Could you check a few things on this model? Use its own coordinates, in mm. A direction names the side the tool comes from. Coordinates: 2 decimals unless noted, no trailing zeros. Loops run counter-clockwise (first coordinate to the right, second up) from the corner with the lowest first, then second, coordinate; pieces in that order, holes last. Notation, with made-up numbers: (-3, 10) - (12, 10) arc R20 cw to (12, 18) - close; hole circle Ø4 at (4.25, 4). An arc over 180 degrees is marked (long way). One line per item, written item: value. Start each with the question number.
(1) If we section it at C-C on y = -6.75: Write out the boundary of the cut face in (x, z).
(2) If we mould it in two halves opening along X, with no side actions, what happens to faces 3 (the face through (-16, -20, 17)), 4 (the face through (-30.092, -9.399, 18.028)), 5 (the face through (-0.285, -19.699, 12.098))? For each: pulls with the +X half, pulls with the -X half, needs draft (parallel to the pull), parting line crosses it, or undercut.
(3) If we section it at D-D on z = 18.5: Write out the boundary of the cut face in (x, y).
(4) If I drill on line 1 along Y through (x, z) = (-32, 19.05); line 2 along X through (y, z) = (-3.25, 7.5); line 3 along Z through (x, y) = (-15, -19), over which ranges is the centre line in solid material (lowest first)? Write a range as from..to.
(5) On a 3-axis mill with a long thin cutter (end or side, diameter ignored), from which of +Z, -Z, +X, -X, +Y, -Y can I reach the whole of each face in a straight line? I mean faces 1 (the face through (-0.285, -10.07, 0.301)), 2 (the face through (-22, -10, 16)). Say none if no direction works.
(6) I'm going to push flat-ended pins straight in: P1, Ø6, axis at x = -23, y = -11.5, coming from the -Z side; P2, Ø10, axis at x = -9.5, z = 4, coming from the -Y side; P3, Ø1.5, axis at y = -3.5, z = 8.5, coming from the -X side. Where does each tip first touch, or does it pass through?
(7) If we section it at A-A on x = -32: Write out the boundary of the cut face in (y, z), then the cut area to 3 significant figures.
(8) If we section it at B-B on z = 8: Write out the boundary of the cut face in (x, y), then the cut area to 3 significant figures.
```python
from build123d import *

# Parameters (mm, degrees)
F1_DEPTH = 20
F2_R     = 2
F3_DEPTH = 25
F4_R     = 2
F5_DEPTH = 25
F6_R     = 5
F7_R     = 1


with BuildPart() as f1:
    # F0 (on Front) → F1 (new body)
    with BuildSketch(Plane.XZ):
        Polygon((-4, 0), (0, 0), (0, 20), (-40, 20), (-40, 16), (-4, 16), align=None)
    extrude(amount=F1_DEPTH)

    # F2 (on face) → F3 (cut)
    with BuildSketch(Plane.XY.offset(20)):
        with Locations((-32, -10)):
            Circle(F2_R)
    extrude(amount=-F3_DEPTH, mode=Mode.SUBTRACT)

    # F4 (on face) → F5 (cut)
    with BuildSketch(Plane.YZ):
        with Locations((-10, 8)):
            Circle(F4_R)
    extrude(amount=-F5_DEPTH, mode=Mode.SUBTRACT)

    # F6
    f6_edges = [f1.edges().sort_by_distance(p)[0] for p in [
        (-2, -20, 0),
        (-2, 0, 0),
        (-40, -20, 18),
        (-40, 0, 18),
    ]]
    fillet(f6_edges, radius=F6_R)

    # F7
    f7_edges = [f1.edges().sort_by_distance(p)[0] for p in [
        (-17.5, -20, 20),
        (0, -20, 12.5),
        (0, -10, 20),
    ]]
    fillet(f7_edges, radius=F7_R)


solid = f1.part
```
Values:
1. outline: (-40, 16) - (-4, 16) - (-4, 0) - (-1, 0) arc R1 ccw to (0, 1) - (0, 19) arc R1 ccw to (-1, 20) - (-39, 20) arc R1 ccw to (-40, 19) - close
2. face 3: needs draft
2. face 4: undercut
2. face 5: pulls with the +X half
3. outline: (-40, -15) arc R5 ccw to (-35, -20) - (-1, -20) arc R1 ccw to (0, -19) - (0, -1) arc R1 ccw to (-1, 0) - (-35, 0) arc R5 ccw to (-40, -5) - close; hole circle Ø4 at (-32, -10)
4. line 1: y = -20..-12, -8..0
4. line 2: x = -4..0
4. line 3: z = 16..20
5. face 1: -Z, +X, +Y, -Y
5. face 2: -Z, -X, +Y, -Y
6. P1: stops at z = 16
6. P2: passes through
6. P3: stops at x = -4
7. outline: (-20, 16) - (-12, 16) - (-12, 20) - (-19, 20) arc R1 ccw to (-20, 19) - close; (-8, 16) - (0, 16) - (0, 19) arc R1 ccw to (-1, 20) - (-8, 20) - close
7. area: 63.6 mm2
8. outline: (-4, -20) - (-1, -20) arc R1 ccw to (0, -19) - (0, -12) - (-4, -12) - close; (-4, -8) - (0, -8) - (0, -1) arc R1 ccw to (-1, 0) - (-4, 0) - close
8. area: 63.6 mm2
